Can you work these out from the model? Positions are in its coordinate system, mm. Face numbers are marked on the shaded views. A direction names the side the tool comes from. Give positions to 0.01 mm unless a question says otherwise; leave off trailing zeros. Order: outer loops, then holes, each group sorted by start corner. A loop starts at its lowest first (then second) coordinate and runs counter-clockwise, first axis right, second up.
Item 1: I want a section at C-C, the plane y = 14.5. Write out the boundary of the cut face in (x, z).
Item 2: Which directions (+Z, -Z, +X, -X, +Y, -Y) give clear straight access to the entire face, cutting with the end or side of a thin tool? Please do the marked faces 1, 2, 3, 4 and 5.
Item 3: I want a section at B-B, the plane z = -9. Write out the boundary of the cut face in (x, y).
Item 4: I want a section at A-A, the plane x = 89. Write out the boundary of the cut face in (y, z).
Item 5: I'm going to push flat-ended pins straight in: pin 1 Ø1 at (y, z) = (5, 1.5) entering from +X; pin 2 Ø1 at (x, z) = (66.5, -5.5) entering from +Y; pin 3 Ø6 at (x, y) = (8.5, 28.5) entering from +Z (3 decimals). Where does each tip first touch, or does it pass through?
Item 6: If I drill on line 1 along Y through (x, z) = (-2.5, 8); line 2 along X through (y, z) = (-4, 4); line 3 along X through (y, z) = (-7.5, 0.5), over which ranges is the centre line in solid material (lowest first)?
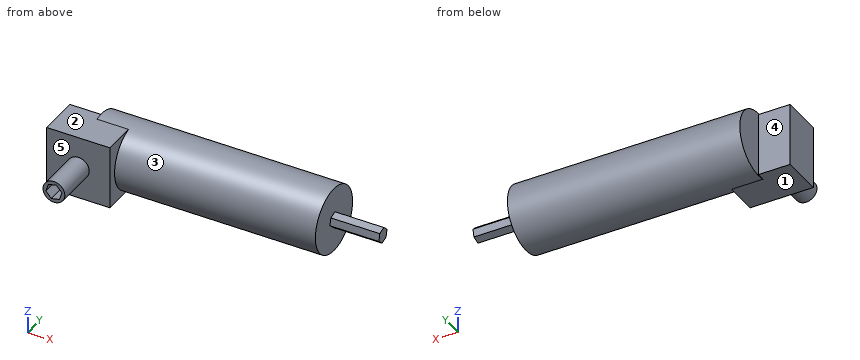
```python
from build123d import *

# Parameters (mm, degrees)
SKETCH1_W           = 31
SKETCH1_H           = 31
BOSS_EXTRUDE1_DEPTH = 20
SKETCH2_R           = 16
BOSS_EXTRUDE2_DEPTH = 114
BOSS_EXTRUDE3_DEPTH = 24
SKETCH4_R           = 5.35
BOSS_EXTRUDE4_DEPTH = 21
CUT_EXTRUDE1_DEPTH  = 7.41


with BuildPart() as part:
    # Sketch1 → Boss-Extrude1 (new body)
    with BuildSketch(Plane(origin=(0, 0, 0), x_dir=(1, 0, 0), z_dir=(0, 1, 0))):
        Rectangle(SKETCH1_W, SKETCH1_H)
    extrude(amount=BOSS_EXTRUDE1_DEPTH)

    # Sketch2 → Boss-Extrude2 (add)
    with BuildSketch(Plane(origin=(0, 0, 0), x_dir=(0, 0, -1), z_dir=(1, 0, 0))):
        with Locations(Location((0, 20, 0), (0, 0, 194.361511563))):
            Circle(SKETCH2_R)
    extrude(amount=BOSS_EXTRUDE2_DEPTH)

    # Sketch3 → Boss-Extrude3 (add)
    with BuildSketch(Plane(origin=(114, 0, 0), x_dir=(0, 0, -1), z_dir=(1, 0, 0))):
        Polygon((2.469779477, 22.709432167), (-1.111547348, 23.493607852), (-3.581326825, 20.784175685), (-2.469779477, 17.290567833), (1.111547348, 16.506392148), (3.581326825, 19.215824315), align=None)
    extrude(amount=BOSS_EXTRUDE3_DEPTH)

    # Sketch4 → Boss-Extrude4 (add)
    with BuildSketch(Plane.XZ):
        with Locations(Location((0, 0, 0), (0, 0, 90))):
            Circle(SKETCH4_R)
    extrude(amount=BOSS_EXTRUDE4_DEPTH)

    # Sketch5 → Cut-Extrude1 (cut)
    with BuildSketch(Plane.XZ.offset(21)):
        Polygon((-3.948474252, -0.861907427), (-1.227803399, -3.850432722), (2.720670854, -2.988525295), (3.948474252, 0.861907427), (1.227803399, 3.850432722), (-2.720670854, 2.988525295), align=None)
    extrude(amount=-CUT_EXTRUDE1_DEPTH, mode=Mode.SUBTRACT)


solid = part.part
```
Results list:
1. outline: (-15.5, -15.5) - (15.5, -15.5) - (15.5, -15.02) - (114, -15.02) - (114, 15.02) - (15.5, 15.02) - (15.5, 15.5) - (-15.5, 15.5) - close
2. face 1: -Z, -X, -Y
2. face 2: +Z, -X, -Y
2. face 3: +X
2. face 4: +Z, -Z, -X, +Y
2. face 5: -Y
3. outline: (-15.5, 0) - (15.5, 0) - (15.5, 6.77) - (114, 6.77) - (114, 33.23) - (0, 33.23) - (0, 20) - (-15.5, 20) - close
4. outline: circle Ø32 at (20, 0)
5. pin 1: stops at x = 114
5. pin 2: stops at y = 35.2
5. pin 3: stops at z = 15.025
6. line 1: y = 0 to 20
6. line 2: x = -3.55 to 3.55
6. line 3: x = -5.33 to 5.33
